For this review, use the dimensioned drawing (mm, ordinates from the lowest corner) and the shaded views. A direction names the side the tool comes from. Coordinates: 2 decimals unless noted, no trailing zeros. Write each loop counter-clockwise with the first axis right and the second up, starting at its lowest first coordinate (ties: lowest second). Pieces come first, ordered by that corner, then holes. Notation, with made-up numbers: (-1.75, 30) -> (45.25, 30) arc R17 ccw to (45.25, 62) -> close; hole circle Ø8 at (34.5, -29). An arc over 180 degrees is marked (long way). Put each result on its own line as item: value. Start each with the question number.
Item 1: Consider section A-A on x = 58. Give the boundary of the cut face in (y, z), and give its area (3 significant figures).
Item 2: Insertion check: P1, Ø5, axis at y = 5, z = 26.5, coming from the +X side; P2, Ø6, axis at y = 10, z = 5.5, coming from the -X side; P3, Ø11.5, axis at x = 63.5, y = 12.7, coming from the -Z side; P4, Ø7.5, axis at y = 17, z = 25, coming from the -X side. Each pin has a flat end and moves straight along its axis. Give the tip position at first contact, or say it passes through.
Item 3: Consider section C-C on x = 33. Give the boundary of the cut face in (y, z), and give its area (3 significant figures).
Item 4: For the marked faces 1 and 2, list the 3-axis set-ups (+Z, -Z, +X, -X, +Y, -Y) from which the entire face can be reached by the end or side of a thin tool; tool diameter is ignored.
Item 5: To check wall thickness, follow L1, parallel to X at y = 12.7, z = 4.75; L2, parallel to Y at x = 63.5, z = 2.5; L3, parallel to Z at x = 32.5, y = 12.7. State the ranges of each line that lie inside material, in increasing order.
Item 6: Consider section D-D on z = 17. Give the boundary of the cut face in (x, y), and give its area (3 significant figures).
Item 7: The part is to be moulded in two halves that separate along X. For the marked faces 3, 4 and 5, say which applies: +X half, -X half, draft (parallel to the pull), parting line (faces both ways), or undercut.
Item 8: Consider section B-B on y = 18. Give the boundary of the cut face in (x, z), and give its area (3 significant figures).
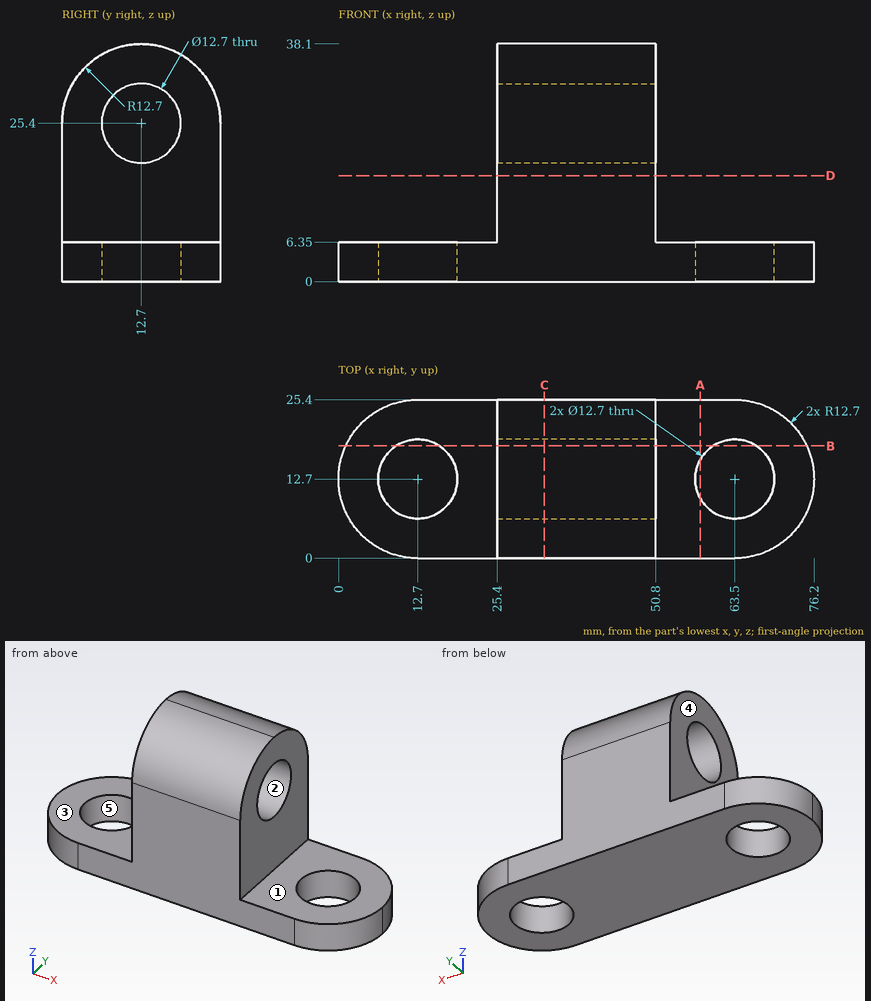
Return value:
1. outline: (0, 0) -> (9.53, 0) -> (9.53, 6.35) -> (0, 6.35) -> close; (15.87, 0) -> (25.4, 0) -> (25.4, 6.35) -> (15.87, 6.35) -> close
1. area: 121 mm^2
2. P1: x = 50.8
2. P2: x = 0
2. P3: through
2. P4: x = 25.4
3. outline: (0, 0) -> (25.4, 0) -> (25.4, 25.4) arc R12.7 ccw to (0, 25.4) -> close; hole circle Ø12.7 at (12.7, 25.4)
3. area: 772 mm^2
4. face 1: +Z, +X, +Y, -Y
4. face 2: +X, -X
5. L1: 0 to 6.35, 19.05 to 57.15, 69.85 to 76.2
5. L2: 0 to 6.35, 19.05 to 25.4
5. L3: 0 to 19.05, 31.75 to 38.1
6. outline: (25.4, 0) -> (50.8, 0) -> (50.8, 25.4) -> (25.4, 25.4) -> close
6. area: 645 mm^2
7. face 3: draft
7. face 4: -X half
7. face 5: undercut
8. outline: (1.16, 0) -> (9.2, 0) -> (9.2, 6.35) -> (1.16, 6.35) -> close; (16.2, 0) -> (60, 0) -> (60, 6.35) -> (50.8, 6.35) -> (50.8, 21.9) -> (25.4, 21.9) -> (25.4, 6.35) -> (16.2, 6.35) -> close; (25.4, 28.9) -> (50.8, 28.9) -> (50.8, 36.94) -> (25.4, 36.94) -> close; (67, 0) -> (75.04, 0) -> (75.04, 6.35) -> (67, 6.35) -> close
8. area: 980 mm^2
